Autodesk Inventor part; units mm, degrees
ref_plane "YZ Plane" through (0, 0, 0) normal (1, 0, 0) x (0, 1, 0)
ref_plane "XZ Plane" through (0, 0, 0) normal (0, 1, 0) x (-1, 0, 0)
ref_plane "XY Plane" through (0, 0, 0) normal (0, 0, 1) x (1, 0, 0)
sketch "Sketch1" plane through (0, 0, 0) normal (0, 0, 1) x (1, 0, 0)
  arc A0 (2.6458, -2.5) -> (-2.6458, -2.5) centre (0, 0.5) ccw
  line L0 (-2.6458, -2.5) -> (2.6458, -2.5)
  arc A1 (-2.8983, -2.4) -> (2.8983, -2.4) centre (0, 0.5) ccw
  line L1 (-2.8983, -2.4) -> (2.8983, -2.4)
  circle A2 centre (0, 0.5) radius 11
  circle A3 centre (0, 0.5) radius 18
  circle A4 centre (0, 0.5) radius 18.1
  circle A5 centre (0, 0) radius 25
  circle A6 centre (0, 0) radius 37.5
  dimension "d0" = 0.1
  dimension "d1" = 0.1
  dimension "d2" = 50
  dimension "d3" = 75
extrude "Extrusion1" add sketch "Sketch1" against normal blind 15 contours L1 A0 | A2
sketch "Sketch3" plane through (0, 0.5, 0) normal (0, 0, 1) x (1, 0, 0)
  circle A0 centre (0, 0) radius 11
  circle A1 centre (0, 0) radius 18
  point P0 (0, -0.5)
extrude "Extrusion2" add sketch "Sketch3" against normal blind 19
sketch "Sketch4" plane through (0, 0.5, 0) normal (0, 0, 1) x (1, 0, 0)
  circle A0 centre (0, 0) radius 18
  circle A1 centre (0, 0) radius 25
  point P0 (0, -0.5)
  dimension "d8" = 50
extrude "Extrusion3" add sketch "Sketch4" against normal blind 45
sketch "Sketch5" plane through (0, 0.5, 0) normal (0, 0, 1) x (1, 0, 0)
  circle A0 centre (0, 0) radius 37.5
  point P0 (0, -0.5)
  dimension "d11" = 75
extrude "Extrusion4" add sketch "Sketch5" along normal blind 5
sketch "Sketch6" plane through (0, 0.5, -45) normal (0, 0, -1) x (-1, 0, 0)
  circle A0 centre (0, 0) radius 37.5
  circle A1 centre (0, 0) radius 18
  point P0 (0, -0.5)
  dimension "d14" = 75
extrude "Extrusion6" add sketch "Sketch6" along normal blind 5
sketch "Sketch8" plane through (0, 0.5, 5) normal (0, 0, 1) x (1, 0, 0)
  arc A0 (2.6458, -3) -> (-2.6458, -3) centre (0, 0) ccw
  line L0 (-2.6458, -3) -> (2.6458, -3)
  circle A1 centre (0, 0) radius 4
  point P0 (0, -0.5)
  point P1 (4, 0)
  point P2 (2.6458, -3)
extrude "Extrusion7" add sketch "Sketch8" along normal blind 6
properties part number "Drum"
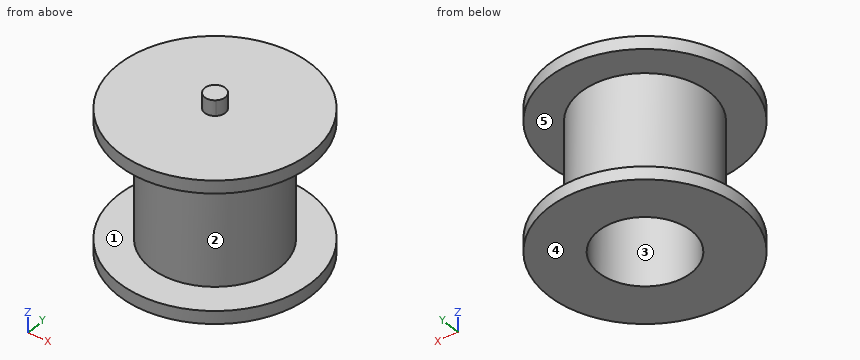
Verification items for the finished model (mm, model axes). Face numbers are marked on the shaded views. A direction names the side the tool comes from. Coordinates: 2 decimals unless noted, no trailing zeros. Write each loop counter-clockwise with the first axis right and the second up, starting at its lowest first coordinate (ties: lowest second). Pieces come first, ordered by that corner, then holes. Notation, with made-up numbers: M 68.5,39.25 L 100.5,39.25 A24 cw 100.5,77.25 Z; hole C -29.5,-37.5 d3. An arc over 180 degrees is marked long. One line per question, with ' | ' between items.
1) Release check for a two-part mould opening along Y. For the marked faces 1, 2 and 3 record: +Y half, -Y half, draft (parallel to the pull), parting line (faces both ways), or undercut.
Solutions:
face 1: draft | face 2: parting line | face 3: undercut
2) Material ranges on L1, parallel to Z at x = 4, y = -31.5; L2, parallel to Y at x = 0, z = -29; L3, parallel to X at y = 0, z = -40 (3 decimals), recorded low to high.
Solutions:
L1: -50 to -45, 0 to 5 | L2: -24.5 to -17.5, 18.5 to 25.5 | L3: -24.995 to -17.993, 17.993 to 24.995
3) Sectioned sample at A-A on x = -32. Record the cut outline in (y, z), then the cut area to 3 significant figures.
Solutions:
outline: M -19.05,-50 L 20.05,-50 L 20.05,-45 L -19.05,-45 Z; M -19.05,0 L 20.05,0 L 20.05,5 L -19.05,5 Z | area: 391 mm^2
4) Access from +Z, -Z, +X, -X, +Y, -Y to the whole of each face (thin tool, end or side, straight path). Record for the marked faces 4 and 5.
Solutions:
face 4: -Z, +X, -X, +Y, -Y | face 5: none
5) Sectioned sample at D-D on x = 0. Record the cut outline in (y, z).
Solutions:
outline: M -37,-50 L -17.5,-50 L -17.5,-19 L -10.5,-19 L -10.5,-15 L -3.6,-15 L -3.6,0 L -2.4,0 L -2.4,-15 L 11.5,-15 L 11.5,-19 L 18.5,-19 L 18.5,-50 L 38,-50 L 38,-45 L 25.5,-45 L 25.5,0 L 38,0 L 38,5 L 4.5,5 L 4.5,11 L -3.5,11 L -3.5,5 L -37,5 L -37,0 L -24.5,0 L -24.5,-45 L -37,-45 Z
6) Sectioned sample at B-B on y = 0.5. Record the cut outline in (x, z).
Solutions:
outline: M -37.5,-50 L -18,-50 L -18,-19 L -11,-19 L -11,-15 L 11,-15 L 11,-19 L 18,-19 L 18,-50 L 37.5,-50 L 37.5,-45 L 25,-45 L 25,0 L 37.5,0 L 37.5,5 L 4,5 L 4,11 L -4,11 L -4,5 L -37.5,5 L -37.5,0 L -25,0 L -25,-45 L -37.5,-45 Z
7) Depth check by flat-ended pin: pin 1 Ø6 at (x, z) = (-24, -32) entering from +Y; pin 2 Ø5 at (y, z) = (4, -9) entering from -X; pin 3 Ø4 at (x, z) = (9, -30.5) entering from -Y. Enter the tip coordinate at first touch or a pass-through.
Solutions:
pin 1: y = 14.06 | pin 2: x = -24.98 | pin 3: y = -23.5
8) Sectioned sample at C-C on z = -20.5. Record the cut outline in (x, y).
Solutions:
outline: C 0,0.5 d50; hole C 0,0.5 d36
